Geometry: final body of the model. Coordinates: model frame, mm. Coordinates: 2 decimals unless noted, no trailing zeros. Loops run counter-clockwise (first coordinate to the right, second up) from the corner with the lowest first, then second, coordinate; pieces in that order, holes last. Notation, with made-up numbers: M 0,70 L 17,70 A18 cw 17,78 Z; hole C 15.25,63 d9. An arc over 180 degrees is marked long. Write item = value, one per line. Start each with the question number.
```python
from build123d import *

# Parameters (mm, degrees)
BASPROSKE_W         = 9
BASPROSKE_H         = 8.125
TOOTHCUT_DEPTH      = 15.595590087
TEETHCUTS_COUNT     = 11
TEETHCUTS_ANGLE     = 327.272727273
BORSKE_R            = 0.5
BORE_DEPTH          = 50.0000508
SKETCH1_R           = 10
BOSS_EXTRUDE1_DEPTH = 3


with BuildPart() as part:
    # BasProSke → Base-Revolve (revolve)
    with BuildSketch(Plane(origin=(0, 0, 0), x_dir=(1, 0, 0), z_dir=(0, 1, 0)), mode=Mode.PRIVATE) as base_revolve_sk:
        with Locations((4.5, 4.0625)):
            Rectangle(BASPROSKE_W, BASPROSKE_H)
    revolve(base_revolve_sk.sketch.rotate(Axis((-10, 0, 0), (1, 0, 0)), 180), axis=Axis((-10, 0, 0), (1, 0, 0)))

    # TooCutSke → ToothCut (cut, through all)
    with BuildSketch(Plane(origin=(0, 0, 0), x_dir=(0, 0, -1), z_dir=(1, 0, 0))):
        with BuildLine():
            ThreePointArc((0.716661614, 5.262929639), (0, 5.3115), (-0.716661614, 5.262929639))
            ThreePointArc((-0.716661614, 5.262929639), (-1.045232485, 6.771828733), (-2.135233901, 7.865735589))
            ThreePointArc((-2.135233901, 7.865735589), (0, 8.1504), (2.135233901, 7.865735589))
            ThreePointArc((2.135233901, 7.865735589), (1.045232485, 6.771828733), (0.716661614, 5.262929639))
        make_face()
    toothcut = extrude(amount=TOOTHCUT_DEPTH, mode=Mode.SUBTRACT)

    # TeethCuts: ToothCut ×11 about axis
    teethcuts_axis = Axis((-10, 0, 0), (1, 0, 0))
    for i in range(1, TEETHCUTS_COUNT):
        add(toothcut.rotate(teethcuts_axis, i * TEETHCUTS_ANGLE / (TEETHCUTS_COUNT - 1)), mode=Mode.SUBTRACT)

    # BorSke → Bore (cut, symmetric)
    with BuildSketch(Plane(origin=(0, 0, 0), x_dir=(0, 0, -1), z_dir=(1, 0, 0))):
        with Locations(Location((0, 0, 0), (0, 0, 180))):
            Circle(BORSKE_R)
    extrude(amount=BORE_DEPTH, both=True, mode=Mode.SUBTRACT)

    # Sketch1 → Boss-Extrude1 (add)
    with BuildSketch(Plane(origin=(9, 0, 0), x_dir=(0, 0, -1), z_dir=(1, 0, 0))):
        Circle(SKETCH1_R)
    extrude(amount=BOSS_EXTRUDE1_DEPTH)


solid = part.part
```
Item 1: Pull-direction query (Y, two-part tool) for faces 1 (the cylindrical face through (4.437, -6.795, -0.904)), 2 (the cylindrical face through (10.48, -9.76, 2.17)); classes: released by +Y, released by -Y, zero draft, split by the parting line, or undercut.
Item 2: First-contact query: pin 1 (6 mm diameter, centred on x = 2.5, z = -6, fed in from -Y); pin 2 (2 mm diameter, centred on x = 5.5, y = 0.5, fed in from -Z). Flat tips, straight axial feed; report the tip coordinate or a pass-through.
Item 3: Section query A-A (z = -1.5). Return the cut outline in (x, y).
Item 4: Line query: line 1 (Y direction, x = 3.5, z = 0) (1 decimal); line 2 (X direction, y = -8.75, z = 2.5); line 3 (Z direction, x = 4, y = -7.75). Output: solid intervals per line, ascending. Write a range as from..to.
Item 5: Section query B-B (y = -0.75). Return the cut outline in (x, z), plus the area to 3 significant figures.
Item 6: Section query D-D (y = -8.5). Return the cut outline in (x, z).
Item 7: Section query C-C (y = 8.75). Return the cut outline in (x, z).
Verdict:
q1.face_1 = undercut
q1.face_2 = split by the parting line
q2.pin_1 = -6.94
q2.pin_2 = -8.07
q3.outline = M 0,-5.1 L 9,-5.1 L 9,-9.89 L 12,-9.89 L 12,9.89 L 9,9.89 L 9,7.38 L 0,7.38 Z
q4.line_1 = -8.1..-0.5, 0.5..5.3
q4.line_2 = 9..12
q4.line_3 = -0.5..0.5
q5.outline = M 0,-5.26 L 9,-5.26 L 9,-9.97 L 12,-9.97 L 12,9.97 L 9,9.97 L 9,5.26 L 0,5.26 Z
q5.area = 154 mm2
q6.outline = M 9,-5.27 L 12,-5.27 L 12,5.27 L 9,5.27 Z
q7.outline = M 9,-4.84 L 12,-4.84 L 12,4.84 L 9,4.84 Z
